Answer from the drawing. Dimensions are ordinates in mm from the lowest x, y and z of the part. Give positions to 0.01 mm unless a question says otherwise; leave off trailing zeros. Loops run counter-clockwise (first coordinate to the right, second up) from the corner with the lowest first, then second, coordinate; pieces in that order, holes last.
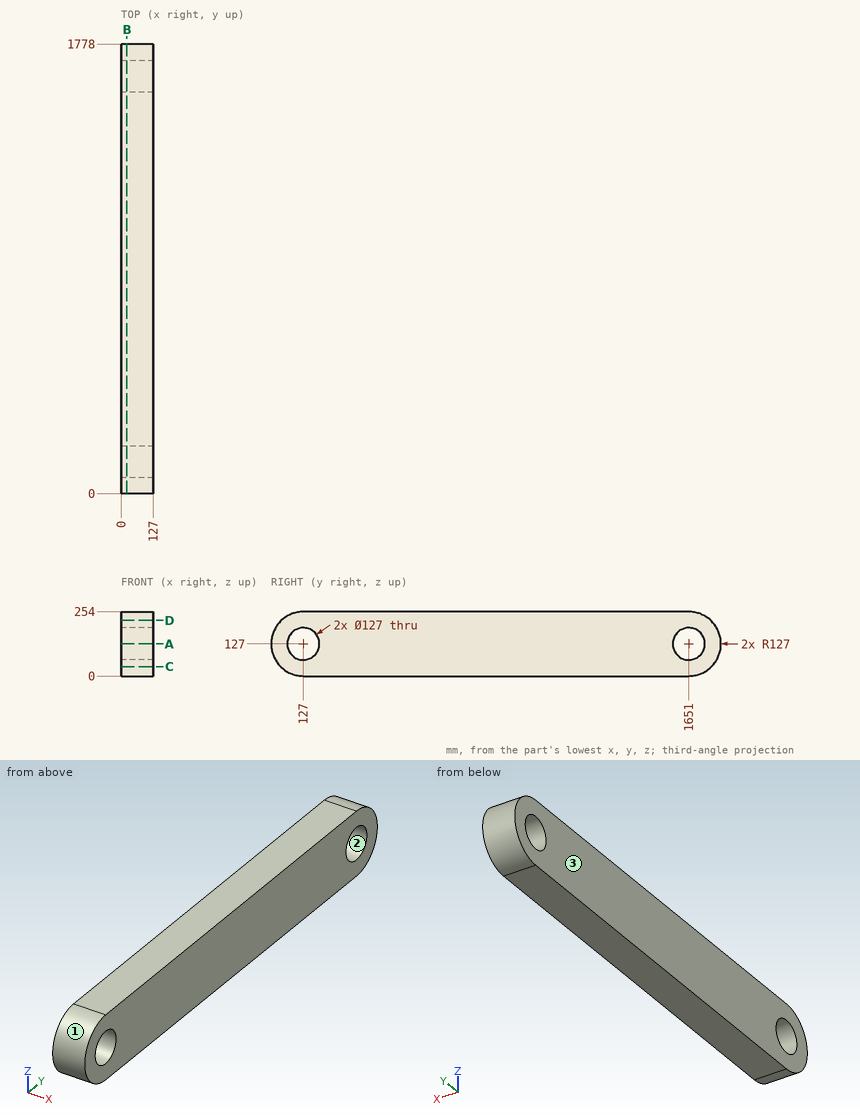
Item 1: Find section D-D, the plane z = 220. Write down the section's boundary in (x, y), plus the area to 3 significant figures.
Item 2: Find section C-C, the plane z = 37. Write down the section's boundary in (x, y).
Item 3: Flat-ended cylindrical pins translate along their axes: pin 1 Ø6 at (x, y) = (36.5, 684) entering from -Z; pin 2 Ø3 at (x, z) = (41.5, 153.5) entering from +Y. Find the tip coordinate at first contact, or state that the pin passes through.
Item 4: Find section B-B, the plane x = 22.5. Write down the section's boundary in (y, z), plus the area to 3 significant figures.
Item 5: Determine the mould class of the marked faces 1, 2 and 3 for opening direction Y: released by +Y, released by -Y, zero draft, split by the parting line, or undercut.
Item 6: Consider line 1 (Y direction, x = 100, z = 160); line 2 (Y direction, x = 42.5, z = 164); line 3 (Z direction, x = 58, y = 127). Determine where each line is inside the solid, lowest interval first.
Item 7: Find section A-A, the plane z = 127. Write down the section's boundary in (x, y), plus the area to 3 significant figures.
Ans:
1. outline: (0, 40.51) - (127, 40.51) - (127, 1737.49) - (0, 1737.49) - close
1. area: 216,000 mm2
2. outline: (0, 37.4) - (127, 37.4) - (127, 1740.6) - (0, 1740.6) - close
3. pin 1: stops at z = 0
3. pin 2: stops at y = 1775.52
4. outline: (127, 0) - (1651, 0) arc R127 ccw to (1651, 254) - (127, 254) arc R127 ccw to start; hole circle Ø127 at (127, 127); hole circle Ø127 at (1651, 127)
4. area: 412,000 mm2
5. face 1: released by -Y
5. face 2: undercut
5. face 3: zero draft
6. line 1: y = 4.36 to 72.75, 181.25 to 1596.75, 1705.25 to 1773.64
6. line 2: y = 5.51 to 75.39, 178.61 to 1599.39, 1702.61 to 1772.49
6. line 3: z = 0 to 63.5, 190.5 to 254
7. outline: (0, 0) - (127, 0) - (127, 63.5) - (0, 63.5) - close; (0, 190.5) - (127, 190.5) - (127, 1587.5) - (0, 1587.5) - close; (0, 1714.5) - (127, 1714.5) - (127, 1778) - (0, 1778) - close
7. area: 194,000 mm2
